Can you work these out from the model? Positions are in its coordinate system, mm. Face numbers are marked on the shaded views. A direction names the side the tool comes from. Round coordinates to 2 decimals unless told otherwise and drop trailing zeros. Write each loop counter-clockwise with the first axis right and the second up, starting at its lowest first coordinate (ties: lowest second). Pieces come first, ordered by that corner, then holes. Notation, with made-up numbers: M 88.5,78 L 98.5,78 A16 cw 98.5,94 Z; hole C 42,28.25 d7. An arc over 180 degrees is marked long. Answer as a JSON object with one key per item and string values. Group by question number.
1) Suppose I cut it at B-B, the plane z = -27.5. Write out the boundary of the cut face in (x, y), and give its area (3 significant figures).
2) I'm going to push flat-ended pins straight in: pin 1 Ø6.5 at (x, z) = (27.5, 0) entering from -Y; pin 2 Ø6 at (x, y) = (-8.5, 10.5) entering from -Z; pin 3 Ø22 at (x, z) = (-7.5, 1.5) entering from -Y; pin 4 Ø4 at (x, z) = (0, 27.5) entering from -Y. Where does each tip first touch, or does it pass through?
3) Suppose I cut it at D-D, the plane y = 2.5. Write out the boundary of the cut face in (x, z).
4) Suppose I cut it at C-C, the plane x = 0. State how many separate pieces and enclosed holes the cut face has, and give its area (3 significant figures).
5) Please list where these lines run through material, in increasing order: L1, parallel to Z at x = 0, y = 14.5; L2, parallel to Y at x = 23, z = 12; L3, parallel to Y at x = 8, z = 13. Write a range as [from, to].
6) On a 3-axis mill with a long thin cutter (end or side, diameter ignored), from which of +Z, -Z, +X, -X, +Y, -Y can I reach the whole of each face in a straight line? I mean the marked faces 5 and 6. Say none if no direction works.
7) Suppose I cut it at A-A, the plane x = -27.5. Write out the boundary of the cut face in (y, z).
8) If we mould it in two halves opening along X, with no side actions, what happens to the marked faces 1, 2, 3 and 4? For each: +X half, -X half, draft (parallel to the pull), parting line (faces both ways), or undercut.
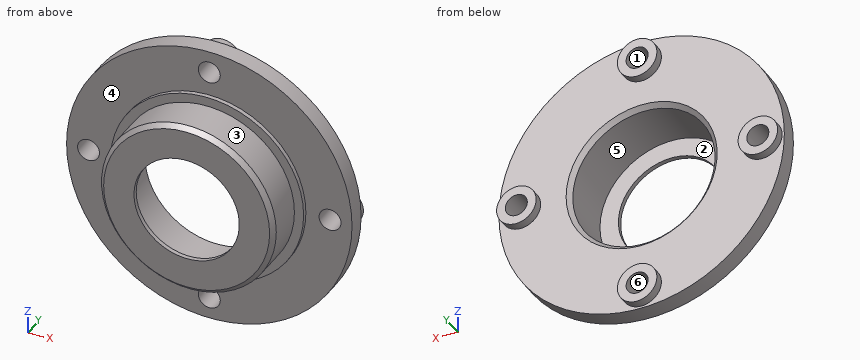
from build123d import *

# Parameters (mm, degrees)
SKETCH1_R           = 19.9
SKETCH1_R_2         = 16.2
BOSS_EXTRUDE1_DEPTH = 9
SKETCH2_R           = 22
SKETCH2_R_2         = 16.2
BOSS_EXTRUDE2_DEPTH = 1
SKETCH3_R           = 32.5
SKETCH3_R_2         = 16.2
BOSS_EXTRUDE3_DEPTH = 1
SKETCH6_R           = 32.5
SKETCH6_R_2         = 2.5
SKETCH6_R_3         = 16.2
BOSS_EXTRUDE6_DEPTH = 3
SKETCH7_R           = 4.5
SKETCH7_R_2         = 2.5
BOSS_EXTRUDE7_DEPTH = 2
SKETCH8_R           = 16.2
SKETCH8_R_2         = 12
BOSS_EXTRUDE8_DEPTH = 1
SKETCH9_R           = 2.5
CUT_EXTRUDE1_DEPTH  = 10
CHAMFER1_SIZE       = 1
CHAMFER2_SIZE       = 1


with BuildPart() as part:
    # Sketch1 → Boss-Extrude1 (new body)
    with BuildSketch(Plane(origin=(0, 0, 0), x_dir=(1, 0, 0), z_dir=(0, 1, 0))):
        Circle(SKETCH1_R)
        Circle(SKETCH1_R_2, mode=Mode.SUBTRACT)
    extrude(amount=BOSS_EXTRUDE1_DEPTH)

    # Sketch2 → Boss-Extrude2 (add)
    with BuildSketch(Plane(origin=(0, 9, 0), x_dir=(1, 0, 0), z_dir=(0, 1, 0))):
        Circle(SKETCH2_R)
        Circle(SKETCH2_R_2, mode=Mode.SUBTRACT)
    extrude(amount=BOSS_EXTRUDE2_DEPTH)

    # Sketch3 → Boss-Extrude3 (add)
    with BuildSketch(Plane(origin=(0, 10, 0), x_dir=(1, 0, 0), z_dir=(0, 1, 0))):
        Circle(SKETCH3_R)
        Circle(SKETCH3_R_2, mode=Mode.SUBTRACT)
    extrude(amount=BOSS_EXTRUDE3_DEPTH)

    # Sketch6 → Boss-Extrude6 (add)
    with BuildSketch(Plane(origin=(0, 11, 0), x_dir=(1, 0, 0), z_dir=(0, 1, 0))):
        Circle(SKETCH6_R)
        with Locations((0, 27.5)):
            Circle(SKETCH6_R_2, mode=Mode.SUBTRACT)
        with Locations((27.5, 0)):
            Circle(SKETCH6_R_2, mode=Mode.SUBTRACT)
        with Locations((0, -27.5)):
            Circle(SKETCH6_R_2, mode=Mode.SUBTRACT)
        with Locations((-27.5, 0)):
            Circle(SKETCH6_R_2, mode=Mode.SUBTRACT)
        Circle(SKETCH6_R_3, mode=Mode.SUBTRACT)
    extrude(amount=BOSS_EXTRUDE6_DEPTH)

    # Sketch7 → Boss-Extrude7 (add)
    with BuildSketch(Plane(origin=(0, 14, 0), x_dir=(1, 0, 0), z_dir=(0, 1, 0))):
        with Locations((0, -27.5)):
            Circle(SKETCH7_R)
        with Locations((0, -27.5)):
            Circle(SKETCH7_R_2, mode=Mode.SUBTRACT)
        with Locations((0, 27.5)):
            Circle(SKETCH7_R)
        with Locations((0, 27.5)):
            Circle(SKETCH7_R_2, mode=Mode.SUBTRACT)
        with Locations((27.5, 0)):
            Circle(SKETCH7_R)
        with Locations((27.5, 0)):
            Circle(SKETCH7_R_2, mode=Mode.SUBTRACT)
        with Locations((-27.5, 0)):
            Circle(SKETCH7_R)
        with Locations((-27.5, 0)):
            Circle(SKETCH7_R_2, mode=Mode.SUBTRACT)
    extrude(amount=BOSS_EXTRUDE7_DEPTH)

    # Sketch8 → Boss-Extrude8 (add)
    with BuildSketch(Plane(origin=(0, 0, 0), x_dir=(-1, 0, 0), z_dir=(0, -1, 0))):
        Circle(SKETCH8_R)
        Circle(SKETCH8_R_2, mode=Mode.SUBTRACT)
    extrude(amount=-BOSS_EXTRUDE8_DEPTH)

    # Sketch9 → Cut-Extrude1 (cut)
    with BuildSketch(Plane(origin=(0, 11, 0), x_dir=(1, 0, 0), z_dir=(0, 1, 0))):
        with Locations((0, -27.5)):
            Circle(SKETCH9_R)
        with Locations((27.5, 0)):
            Circle(SKETCH9_R)
        with Locations((0, 27.5)):
            Circle(SKETCH9_R)
        with Locations((-27.5, 0)):
            Circle(SKETCH9_R)
    extrude(amount=-CUT_EXTRUDE1_DEPTH, mode=Mode.SUBTRACT)

    # Chamfer1
    chamfer1_edges = [part.edges().sort_by_distance(p)[0] for p in [
        (-16.2, 14, 0),
    ]]
    chamfer(chamfer1_edges, length=CHAMFER1_SIZE)

    # Chamfer2
    chamfer2_edges = [part.edges().sort_by_distance(p)[0] for p in [
        (-19.9, 0, 0),
    ]]
    chamfer(chamfer2_edges, length=CHAMFER2_SIZE)


solid = part.part
Results:
{
 "1": {"outline": "M -17.32,10 L -2.5,10 L -2.5,16 L -4.5,16 L -4.5,14 L -17.32,14 Z; M 2.5,10 L 17.32,10 L 17.32,14 L 4.5,14 L 4.5,16 L 2.5,16 Z", "area": "127 mm^2"},
 "2": {"pin 1": "y = 10", "pin 2": "z = -32.03", "pin 3": "y = 0", "pin 4": "through"},
 "3": {"outline": "C 0,0 d39.8; hole C 0,0 d32.4"},
 "4": {"separate pieces": "4", "enclosed holes": "0", "area": "191 mm^2"},
 "5": {"L1": "[-32, -30], [-25, -23], [23, 25], [30, 32]", "L2": "[10, 14]", "L3": "[0, 1]"},
 "6": {"face 5": "+Y", "face 6": "+Y, -Y"},
 "7": {"outline": "M 10,-17.32 L 14,-17.32 L 14,-4.5 L 16,-4.5 L 16,-2.5 L 10,-2.5 Z; M 10,2.5 L 16,2.5 L 16,4.5 L 14,4.5 L 14,17.32 L 10,17.32 Z"},
 "8": {"face 1": "undercut", "face 2": "undercut", "face 3": "parting line", "face 4": "draft"}
}
